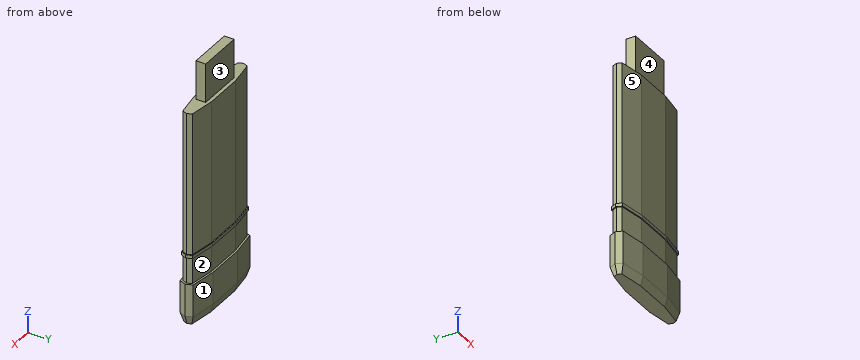
```python
from build123d import *

# Parameters (mm, degrees)
F1_DEPTH  = 63.5
F4_DEPTH  = 17.78
F4_TAPER  = 17
F6_DEPTH  = 50.8
F8_DEPTH  = 6.35
F10_DEPTH = 279.4
F11_W     = 88.9
F11_H     = 19.05
F12_DEPTH = 76.2


with BuildPart() as f1:
    # F0 (on Top) → F1 (new body)
    with BuildSketch(Plane.XY):
        Polygon((-57.5468856689, 20.32), (-108.3468856689, 12.7), (-113.5062576618, 0), (-108.4262576618, -12.7), (-57.5468856689, -20.32), (18.6531143311, -20.32), (69.4531143311, -12.7), (74.5331143311, 0), (69.4531143311, 12.7), (18.6531143311, 20.32), align=None)
    extrude(amount=F1_DEPTH)

    # F3 (on face) → F4 (join)
    with BuildSketch(Plane(origin=(0, 0, 0), x_dir=(1, 0, 0), z_dir=(0, 0, -1))):
        Polygon((-113.5062576618, 0), (-108.3468856689, -12.7), (-57.5468856689, -20.32), (18.6531143311, -20.32), (69.4531143311, -12.7), (74.5331143311, 0), (69.4531143311, 12.7), (18.6531143311, 20.32), (-57.5468856689, 20.32), (-108.4262576618, 12.7), align=None)
        Polygon((-56.9794414883, 12.7), (18.0847933541, 12.7), (64.0011016636, 5.8125537536), (66.326123165, 0), (64.0011016636, -5.8125537536), (18.0847933541, -12.7), (-56.9785646919, -12.7), (-102.921750061, -5.8085221946), (-105.2904326731, 0.0220845566), (-102.9746753651, 5.8114778266), align=None, mode=Mode.SUBTRACT)
        Polygon((64.0011016636, 5.8125537536), (18.0847933541, 12.7), (-56.9794414883, 12.7), (-102.9746753651, 5.8114778266), (-105.2904326731, 0.0220845566), (-102.921750061, -5.8085221946), (-56.9785646919, -12.7), (18.0847933541, -12.7), (64.0011016636, -5.8125537536), (66.326123165, 0), align=None)
    extrude(amount=F4_DEPTH, taper=F4_TAPER)

    # F5 (on face) → F6 (join)
    with BuildSketch(Plane.XY.offset(63.5)):
        Polygon((-105.634317865, 9.2542610973), (-109.3983451675, -0.0110422783), (-105.7004665135, -9.2557389133), (-57.2631635786, -16.51), (18.3689538426, -16.51), (66.7271079974, -9.2562768768), (70.4296187481, 0), (66.7271079974, 9.2562768768), (18.3689538426, 16.51), (-57.2627251804, 16.51), align=None)
    extrude(amount=F6_DEPTH)

    # F7 (on face) → F8 (join)
    with BuildSketch(Plane.XY.offset(114.3)):
        Polygon((-57.4050246237, -18.415), (18.5110340868, -18.415), (68.0901111642, -10.9781384384), (72.4813665396, 0), (68.0901111642, 10.9781384384), (18.5110340868, 18.415), (-57.4048054246, 18.415), (-106.9906017669, 10.9771305487), (-111.4523014147, -0.0055211391), (-107.0633620877, -10.9778694567), align=None)
    extrude(amount=F8_DEPTH)

    # F9 (on face) → F10 (join)
    with BuildSketch(Plane.XY.offset(120.65)):
        Polygon((70.4296187481, 0), (66.7271079974, 9.2562768768), (18.3689538426, 16.51), (-57.2627251804, 16.51), (-105.634317865, 9.2542610973), (-109.3983451675, -0.0110422783), (-105.7004665135, -9.2557389133), (-57.2631635786, -16.51), (18.3689538426, -16.51), (66.7271079974, -9.2562768768), align=None)
    extrude(amount=F10_DEPTH)

    # F11 (on face) → F12 (join)
    with BuildSketch(Plane.XY.offset(400.05)):
        with Locations((-19.4468856689, -0.0110422783)):
            Rectangle(F11_W, F11_H)
    extrude(amount=F12_DEPTH)


solid = f1.part
```
Work out the finished part from the listing and answer in its coordinate system (mm). Face numbers are marked on the shaded views. A direction names the side the tool comes from. Round coordinates to 2 decimals unless told otherwise and drop trailing zeros. Write each loop counter-clockwise with the first axis right and the second up, starting at its lowest first coordinate (ties: lowest second). Pieces come first, ordered by that corner, then holes.
1) Which of the six approach directions +Z, -Z, +X, -X, +Y, -Y give full straight-line access (tool end or side, diameter ignored) to the marked faces 3, 4 and 5?
2) Consider probe 1 along X at (y, z) = (0, 456); probe 2 along Z at (x, y) = (38, 10); probe 3 along Y at (x, z) = (64.5, 261.5). Determine where each line is inside the solid, lowest interval first.
3) A cutting plane is placed at B-B on z = 442. Determine the outline of the cut face in (x, y).
4) A cutting plane is placed at A-A on z = 272. Determine the outline of the cut face in (x, y).
5) Flat-ended cylindrical pins translate along their axes: P1, Ø5, axis at x = 9, z = 364, coming from the -Y side; P2, Ø21, axis at y = 1.5, z = 424, coming from the +X side; P3, Ø15, axis at y = 0, z = 430.5, coming from the -X side. Find the tip coordinate at first contact, or state that the pin passes through.
6) Determine the mould class of the marked faces 1 and 2 for opening direction Z: pulls with the +Z half, pulls with the -Z half, needs draft (parallel to the pull), parting line crosses it, or undercut.
Entries:
1. face 3: +Z, +X, -X, +Y
1. face 4: +Z, +X, -X, -Y
1. face 5: +Z, -X, -Y
2. probe 1: x = -63.9 to 25
2. probe 2: z = -17.78 to 400.05
2. probe 3: y = -9.59 to 9.59
3. outline: (-63.9, -9.54) - (25, -9.54) - (25, 9.51) - (-63.9, 9.51) - close
4. outline: (-109.4, -0.01) - (-105.7, -9.26) - (-57.26, -16.51) - (18.37, -16.51) - (66.73, -9.26) - (70.43, 0) - (66.73, 9.26) - (18.37, 16.51) - (-57.26, 16.51) - (-105.63, 9.25) - close
5. P1: stops at y = -16.51
5. P2: stops at x = 25
5. P3: stops at x = -63.9
6. face 1: needs draft
6. face 2: undercut
